Model file for the job. Use its own axes, mm. A direction names the side the tool comes from. Give positions to 0.01 mm unless a question says otherwise; leave off trailing zeros. Write each loop counter-clockwise with the first axis right and the second up, starting at its lowest first coordinate (ties: lowest second). Pieces come first, ordered by that corner, then holes.
Autodesk Inventor part; units mm, degrees
ref_plane "YZ Plane" through (0, 0, 0) normal (1, 0, 0) x (0, 1, 0)
ref_plane "XZ Plane" through (0, 0, 0) normal (0, 1, 0) x (-1, 0, 0)
ref_plane "XY Plane" through (0, 0, 0) normal (0, 0, 1) x (1, 0, 0)
sketch "Sketch1" plane through (0, 0, 0) normal (0, 0, 1) x (1, 0, 0)
  arc A0 (-19.9373, 1) -> (-4.0627, 1) centre (-12, 0) ccw
  arc A1 (4.0627, 1) -> (19.9373, 1) centre (12, 0) ccw
  line L0 (0, 1) -> (-4.0627, 1)
  line L1 (0, 1) -> (4.0627, 1)
  line L2 (-24, 0) -> (-24, 1)
  line L3 (-19.9373, 1) -> (-24, 1)
  line L4 (24, 0) -> (24, 1)
  line L5 (24, 1) -> (19.9373, 1)
  line L6 (24, 0) -> (24, -12)
  line L7 (24, -12) -> (-24, -12)
  line L8 (-24, -12) -> (-24, 0)
  line L9 (24, 1) -> (24, -12)
  line L10 (24, -12) -> (-24, -12)
  line L11 (-24, -12) -> (-24, 1)
  line L12 (-24, 1) -> (-19.9373, 1)
  line L13 (-4.0627, 1) -> (4.0627, 1)
  line L14 (19.9373, 1) -> (24, 1)
  point P0 (0, 0)
  dimension "d4" = 12
  dimension "d5" = 12
  dimension "d6" = 1
  dimension "d7" = 12
extrude "Extrusion1" add sketch "Sketch1" along normal blind 9.5
sketch "Sketch2" plane through (-24, -12, 0) normal (0, -1, 0) x (1, 0, 0)
  line L0 (0, 9.5) -> (48, 9.5)
  line L1 (0, 9.5) -> (48, 9.5)
  line L2 (48, 9.5) -> (48, -20.5)
  line L3 (48, -20.5) -> (0, -20.5)
  line L4 (0, -20.5) -> (0, 9.5)
  point P0 (24, 0)
  dimension "d10" = 30
extrude "Extrusion2" add sketch "Sketch2" along normal blind 2
sketch "Sketch3" plane through (-24, -14, 0) normal (0, -1, 0) x (1, 0, 0)
  line L0 (48, 9.5) -> (0, 9.5)
  line L1 (0, 9.5) -> (0, -20.5)
  line L2 (0, -20.5) -> (48, -20.5)
  line L3 (48, -20.5) -> (48, 9.5)
  point P0 (24, 0)
revolve "Revolution1" add sketch "Sketch3" angle 15 about axis through (24, -14, 9.5) along (-1, 0, 0)
sketch "Sketch4" plane through (-24, -14, 9.5) normal (0, -0.9659, 0.2588) x (1, 0, 0)
  line L0 (48, -28.9778) -> (48, -30)
  line L1 (48, -30) -> (0, -30)
  line L2 (0, -30) -> (0, -15)
  line L3 (48, -15) -> (48, -30)
  line L4 (48, -8.6587) -> (48, -28.4601)
  line L5 (0, -28.4601) -> (0, -8.6587)
  arc A0 (48, -15) -> (0, -15) centre (24, -70.1) ccw
  point P0 (24, -5.5528)
extrude "Extrusion3" add sketch "Sketch4" along normal blind 12
sketch "Sketch5" plane through (-24, -25.5911, 12.6058) normal (0, -0.9659, 0.2588) x (1, 0, 0)
  arc A0 (48, -15) -> (0, -15) centre (24, -70.1) ccw
  arc A1 (48, -15) -> (0, -15) centre (24, -70.1) ccw
  line L0 (48, -15) -> (48, -40)
  line L1 (0, -15) -> (0, -40)
  line L2 (0, -40) -> (48, -40)
  point P0 (24, -5.5528)
  dimension "d19" = 25
  dimension "d20" = 25
extrude "Extrusion4" add sketch "Sketch5" along normal blind 2
properties part number "HatSensorMount02FB"
1. Pull direction X, two halves, no side cores. Call faces 6 (the flat face through (-0.34, -33.94, -10.82)), 7 (the cylindrical face through (-0.35, -22.3, 1.37)), 8 (the cylindrical face through (-12, -8, 5)): +X half, -X half, draft (parallel to the pull), parting line (faces both ways), or undercut.
Calculated:
face 6: draft
face 7: parting line
face 8: undercut
2. Slice it at B-B, the plane z = -17.5. Write the cut outline in (x, y).
Calculated:
outline: (-24, -35.73) - (24, -35.73) - (24, -33.66) - (-24, -33.66) - close; (-24, -29.15) - (24, -29.15) - (24, -12) - (-24, -12) - close
3. Pin check, flat tips, straight feed: P1, Ø1, axis at x = -6, y = -12.5, coming from the -Z side; P2, Ø14.5, axis at x = 0, y = -4.5, coming from the -Z side; P3, Ø1, axis at x = -4.5, z = -6.5, coming from the +Y side; P4, Ø12, axis at y = -23, z = 2, coming from the -X side. Stop position of each tip, or through.
Calculated:
P1: stops at z = -20.5
P2: stops at z = 0
P3: stops at y = -12
P4: stops at x = -24
4. Slice it at D-D, the plane y = -7. Write the cut outline in (x, z), and give its area (3 significant figures).
Calculated:
outline: (-24, 0) - (-15.87, 0) - (-15.87, 9.5) - (-24, 9.5) - close; (-8.13, 0) - (8.13, 0) - (8.13, 9.5) - (-8.13, 9.5) - close; (15.87, 0) - (24, 0) - (24, 9.5) - (15.87, 9.5) - close
area: 309 mm2
5. Which spindle directions (+Z, -Z, +X, -X, +Y, -Y) get a long thin tool onto all of the face, cutting with end or side? Do faces 1 (the flat face through (0, -13, -20.5)), 2 (the cylindrical face through (-0.35, -29.13, 3.2)), 3 (the flat face through (22, 1, 5)), 4 (the cylindrical face through (12, -8, 5)), 5 (the cylindrical face through (0.336, -17.97, -20.236)). Say none if no direction does.
Calculated:
face 1: -Z, +X, -X, +Y
face 2: +Z
face 3: +Z, -Z, +X, -X, +Y
face 4: +Z, -Z
face 5: -Z, +X, -X
6. Slice it at A-A, the plane y = 0. Write the cut outline in (x, z).
Calculated:
outline: (-24, 0) - (-20, 0) - (-20, 9.5) - (-24, 9.5) - close; (-4, 0) - (4, 0) - (4, 9.5) - (-4, 9.5) - close; (20, 0) - (24, 0) - (24, 9.5) - (20, 9.5) - close
7. Probe probe 1 along X at (y, z) = (0, 7); probe 2 along Z at (x, y) = (-18, -13); probe 3 along X at (y, z) = (-3, 0.5). List the from-to ranges inside material, lowest first.
Calculated:
probe 1: x = -24 to -20, -4 to 4, 20 to 24
probe 2: z = -20.5 to 9.5
probe 3: x = -24 to -19.42, -4.58 to 4.58, 19.42 to 24
